from build123d import *

# Parameters (mm, degrees)
F0_R     = 22.41
F0_R_2   = 20.94
F0_R_3   = 19.5
F0_R_4   = 9.87
F1_DEPTH = 4
F2_DEPTH = 7


with BuildPart() as f1:
    # F0 (on Top) → F1 (new body)
    with BuildSketch(Plane.XY):
        Circle(F0_R)
        Circle(F0_R_2, mode=Mode.SUBTRACT)
        Circle(F0_R_2)
        Circle(F0_R_3, mode=Mode.SUBTRACT)
        Circle(F0_R_3)
        Circle(F0_R_4, mode=Mode.SUBTRACT)
    extrude(amount=F1_DEPTH)

    # F0 (on Top) → F2 (join)
    with BuildSketch(Plane.XY):
        Circle(F0_R_2)
        Circle(F0_R_3, mode=Mode.SUBTRACT)
    extrude(amount=F2_DEPTH)


solid = f1.part
Model file for the job. Use its own axes, mm. A direction names the side the tool comes from. Give positions to 0.01 mm unless a question says otherwise; leave off trailing zeros. Order: outer loops, then holes, each group sorted by start corner. A loop starts at its lowest first (then second) coordinate and runs counter-clockwise, first axis right, second up. Notation, with made-up numbers: (-7.75, 74) - (42.25, 74) arc R24 ccw to (42.25, 97) - close; hole circle Ø11 at (39, -0.5). An arc over 180 degrees is marked (long way). Write item = value, one per line. Start each with the question number.
1. Cut at C-C, the plane z = 6. List the corners of the cut face in (x, y).
2. Which spindle directions (+Z, -Z, +X, -X, +Y, -Y) get a long thin tool onto all of the face, cutting with end or side? Do faces 4 (the cylindrical face through (19.973, 6.29, 5.479)), 5 (the flat face through (19, 6, 7)). Say none if no direction does.
3. Drop flat-ended pins along their axis: P1, Ø2, axis at x = -8.5, z = 2, coming from the +Y side; P2, Ø2, axis at x = 5, y = 12, coming from the +Z side; P3, Ø1.5, axis at y = -2.5, z = 2.5, coming from the -X side. Give the stop position or say it passes through.
4. Cut at D-D, the plane y = 17. List the corners of the cut face in (x, z), and give its area (3 significant figures).
5. Cut at A-A, the plane x = 0. List the corners of the cut face in (y, z).
6. Two-plate mould, pull along X, no slides. Class faces 1 (the cylindrical face through (-2.14, -9.635, 1.972)), 2 (the flat face through (10, -5, 0)), 3 (the cylindrical face through (21.375, 6.731, 1.972)): pulls with the +X half, pulls with the -X half, needs draft (parallel to the pull), parting line crosses it, or undercut.
7. Probe line 1 along Y through (x, z) = (0, 5.7); line 2 along Y through (x, z) = (0, 1). List the from-to ranges inside material, lowest first.
Taken from the geometry:
q1.outline = circle Ø41.88 at (0, 0); hole circle Ø39 at (0, 0)
q2.face_4 = +Z
q2.face_5 = +Z, +X, -X, +Y, -Y
q3.P1 = 21.12
q3.P2 = 4
q3.P3 = -22.34
q4.outline = (-14.6, 0) - (14.6, 0) - (14.6, 4) - (12.23, 4) - (12.23, 7) - (9.55, 7) - (9.55, 4) - (-9.55, 4) - (-9.55, 7) - (-12.23, 7) - (-12.23, 4) - (-14.6, 4) - close
q4.area = 133 mm²
q5.outline = (-22.41, 0) - (-9.87, 0) - (-9.87, 4) - (-19.5, 4) - (-19.5, 7) - (-20.94, 7) - (-20.94, 4) - (-22.41, 4) - close; (9.87, 0) - (22.41, 0) - (22.41, 4) - (20.94, 4) - (20.94, 7) - (19.5, 7) - (19.5, 4) - (9.87, 4) - close
q6.face_1 = undercut
q6.face_2 = needs draft
q6.face_3 = parting line crosses it
q7.line_1 = -20.94 to -19.5, 19.5 to 20.94
q7.line_2 = -22.41 to -9.87, 9.87 to 22.41
